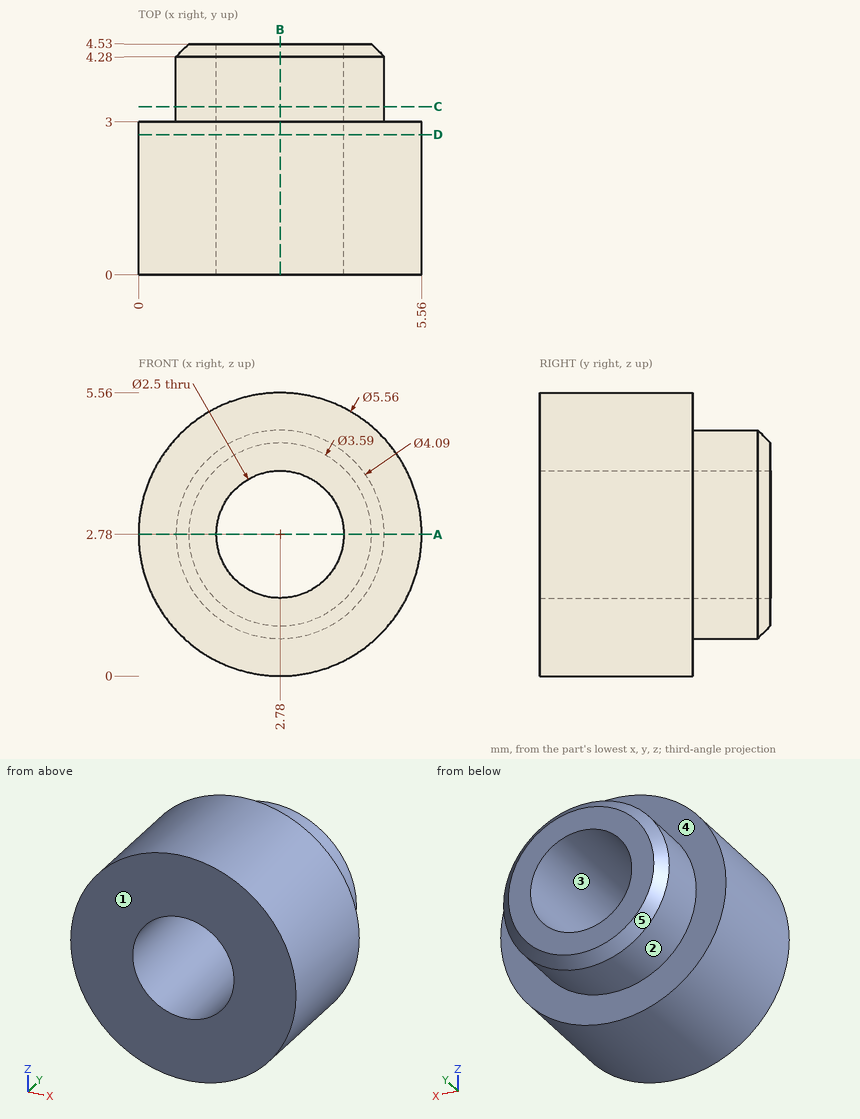
Check sheet for the drawn part. Datum: minimum x, y, z corner. Units: mm. A direction names the side the tool comes from. Round coordinates to 2 decimals unless told otherwise and drop trailing zeros. Write each loop counter-clockwise with the first axis right and the second up, starting at its lowest first coordinate (ties: lowest second). Pieces come first, ordered by that corner, then holes. Notation, with made-up numbers: (62.5, -26) -> (108.5, -26) arc R15 ccw to (108.5, -6) -> close; hole circle Ø11 at (79, 58.5). An arc over 180 degrees is marked (long way). One line per item, written item: value. Start each with the question number.
(1) Draft check along X on the marked faces 3, 4 and 5. Enter one of: +X half, -X half, draft (parallel to the pull), parting line (faces both ways), or undercut.
(2) Cross-section at B-B, the plane x = 2.78. Record the cut outline in (y, z) (3 decimals).
(3) Cross-section at A-A, the plane z = 2.78. Record the cut outline in (x, y) (3 decimals).
(4) Go/stop test with a flat-tipped pin: pin 1 Ø2 at (x, z) = (1.5, 4) entering from -Y. Record where the tip stops, or that it passes through.
(5) Cross-section at C-C, the plane y = 3.3. Record the cut outline in (x, z) (3 decimals).
(6) Cross-section at D-D, the plane y = 2.75. Record the cut outline in (x, z).
(7) Scan lines: line 1 (Z direction, x = 2.78, y = 2.1); line 2 (Z direction, x = 2.78, y = 3.45) (3 decimals); line 3 (Y direction, x = 4.75, z = 4.4). Record each from-to range of solid material in increasing order. Write a range as [from, to].
(8) Access from +Z, -Z, +X, -X, +Y, -Y to the whole of each face (thin tool, end or side, straight path). Record for the marked faces 1 and 2.
Answer:
1. face 3: undercut
1. face 4: draft
1. face 5: parting line
2. outline: (0, 0) -> (3, 0) -> (3, 0.735) -> (4.28, 0.735) -> (4.53, 0.985) -> (4.53, 1.53) -> (0, 1.53) -> close; (0, 4.03) -> (4.53, 4.03) -> (4.53, 4.575) -> (4.28, 4.825) -> (3, 4.825) -> (3, 5.56) -> (0, 5.56) -> close
3. outline: (0, 0) -> (1.53, 0) -> (1.53, 4.53) -> (0.985, 4.53) -> (0.735, 4.28) -> (0.735, 3) -> (0, 3) -> close; (4.03, 0) -> (5.56, 0) -> (5.56, 3) -> (4.825, 3) -> (4.825, 4.28) -> (4.575, 4.53) -> (4.03, 4.53) -> close
4. pin 1: y = 0
5. outline: circle Ø4.09 at (2.78, 2.78); hole circle Ø2.5 at (2.78, 2.78)
6. outline: circle Ø5.56 at (2.78, 2.78); hole circle Ø2.5 at (2.78, 2.78)
7. line 1: [0, 1.53], [4.03, 5.56]
7. line 2: [0.735, 1.53], [4.03, 4.825]
7. line 3: [0, 3]
8. face 1: +Z, -Z, +X, -X, -Y
8. face 2: +Y
